```python
from build123d import *

# Parameters (mm, degrees)
F0_W     = 190.5
F0_H     = 50.8
F1_DEPTH = 50.8
F2_W     = 45.588648
F2_H     = 45.72
F3_DEPTH = 237.56619


with BuildPart() as f1:
    # F0 (on Top) → F1 (new body)
    with BuildSketch(Plane.XY):
        Rectangle(F0_W, F0_H)
    extrude(amount=F1_DEPTH)

    # F2 (on face) → F3 (cut)
    with BuildSketch(Plane.YZ.offset(95.25)):
        with Locations((0, 25.4)):
            Rectangle(F2_W, F2_H)
    extrude(amount=-F3_DEPTH, mode=Mode.SUBTRACT)


solid = f1.part
```
The listing builds one solid part. Answer for the finished solid, in the listing's coordinates (mm). A direction names the side the tool comes from. Round coordinates to 2 decimals unless told otherwise and drop trailing zeros. Loops run counter-clockwise (first coordinate to the right, second up) from the corner with the lowest first, then second, coordinate; pieces in that order, holes last.
1) A cutting plane is placed at B-B on y = 18. Determine the outline of the cut face in (x, z), plus the area to 3 significant figures.
Outcome:
outline: (-95.25, 0) - (95.25, 0) - (95.25, 2.54) - (-95.25, 2.54) - close; (-95.25, 48.26) - (95.25, 48.26) - (95.25, 50.8) - (-95.25, 50.8) - close
area: 968 mm2
2) A cutting plane is placed at A-A on z = 45.5. Determine the outline of the cut face in (x, y), plus the area to 3 significant figures.
Outcome:
outline: (-95.25, -25.4) - (95.25, -25.4) - (95.25, -22.79) - (-95.25, -22.79) - close; (-95.25, 22.79) - (95.25, 22.79) - (95.25, 25.4) - (-95.25, 25.4) - close
area: 993 mm2
3) For faces 4 (the face through (1, -22.794, 25)), 5 (the face through (-1, 0, 0)), determine the directions among +Z, -Z, +X, -X, +Y, -Y from which every point of the face is accessible in a straight line to the end or side of a thin tool.
Outcome:
face 4: +X, -X
face 5: -Z, +X, -X, +Y, -Y
4) Consider line 1 (Y direction, x = 9, z = 19.5); line 2 (Z direction, x = -68, y = 1). Determine where each line is inside the solid, lowest interval first.
Outcome:
line 1: y = -25.4 to -22.79, 22.79 to 25.4
line 2: z = 0 to 2.54, 48.26 to 50.8
5) A cutting plane is placed at C-C on x = 18. Determine the outline of the cut face in (y, z).
Outcome:
outline: (-25.4, 0) - (25.4, 0) - (25.4, 50.8) - (-25.4, 50.8) - close; hole (-22.79, 2.54) - (22.79, 2.54) - (22.79, 48.26) - (-22.79, 48.26) - close
6) For a pull along Y with two mould halves and no side action, classify faces 1 (the face through (1, 22.794, 25)), 2 (the face through (-1, 0, 50.8)), 3 (the face through (-1, 25.4, 25)) as released by +Y, released by -Y, zero draft, split by the parting line, or undercut.
Outcome:
face 1: undercut
face 2: zero draft
face 3: released by +Y
